Part model, mm, in its own coordinate system. Round coordinates to 2 decimals unless told otherwise and drop trailing zeros. Write each loop counter-clockwise with the first axis right and the second up, starting at its lowest first coordinate (ties: lowest second). Pieces come first, ordered by that corner, then holes. Notation, with made-up numbers: (-19.75, -31) -> (28.25, -31) arc R15 ccw to (28.25, -16) -> close; hole circle Ø10 at (82.5, -6.75). An arc over 180 degrees is marked (long way). Use CSV: the item, a comma, the result in double quotes. Start each with the question number.
(1) Probe line 1 (Z direction, x = 17.5, y = 41); line 2 (Y direction, x = 14.5, z = 15); line 3 (Y direction, x = 12.25, z = 35). List the from-to ranges inside material, lowest first. Write a range as [from, to].
(2) Saw through at D-D (y = 30.5). Give the cut face in (x, z).
(3) Saw through at C-C (y = 42.5). Count the separate pieces of the cut face and the enclosed holes in it, plus the area to 3 significant figures.
(4) Two-plate mould, pull along Z, no slides. Class faces 1 (the flat face through (10, 65, 25)), 2 (the flat face through (12, 33, 0)), 3 (the cylindrical face through (9.63, 44.47, 15.52)): released by +Z, released by -Z, zero draft, split by the parting line, or undercut.
(5) Saw through at B-B (z = 41.5). Give the cut face in (x, y), plus the area to 3 significant figures.
(6) Saw through at A-A (z = 15). Give the cut face in (x, y).
(7) Drop flat-ended pins along their axis: pin 1 (4 mm diameter, centred on y = 57, z = 27.5, fed in from -X); pin 2 (1 mm diameter, centred on y = 29, z = 18, fed in from -X). Give the stop position or say it passes through.
```python
from build123d import *

# Parameters (mm, degrees)
BOSS_EXTRUDE1_DEPTH = 50
SKETCH2_R           = 4
CUT_EXTRUDE1_DEPTH  = 20
CHAMFER1_SIZE       = 1


with BuildPart() as part:
    # Sketch1 → Boss-Extrude1 (new body)
    with BuildSketch(Plane.XY):
        with BuildLine():
            Line((0, 0), (20, 0))
            Line((20, 0), (20, 65))
            Line((20, 65), (0, 65))
            Line((0, 65), (0, 61.14955156))
            ThreePointArc((0, 61.14955156), (6.5, 53.716517187), (0, 46.283482813))
            Line((0, 46.283482813), (0, 33.716517187))
            ThreePointArc((0, 33.716517187), (14, 18.74988764), (0, 3.783258093))
            Line((0, 3.783258093), (0, 0))
        make_face()
    extrude(amount=BOSS_EXTRUDE1_DEPTH)

    # Sketch2 → Cut-Extrude1 (cut)
    with BuildSketch(Plane(origin=(20, 0, 0), x_dir=(0, 0, -1), z_dir=(1, 0, 0))):
        with Locations((-35, 40.505102572)):
            Circle(SKETCH2_R)
        with Locations((-15, 40.505102572)):
            Circle(SKETCH2_R)
    extrude(amount=-CUT_EXTRUDE1_DEPTH, mode=Mode.SUBTRACT)

    # Chamfer1
    chamfer1_edges = [part.edges().sort_by_distance(p)[0] for p in [
        (20, 40.505102572, 39),
        (20, 40.505102572, 19),
    ]]
    chamfer(chamfer1_edges, length=CHAMFER1_SIZE)


solid = part.part
```
Answers:
1,line 1,"z = [0, 11.03], [18.97, 31.03], [38.97, 50]"
1,line 2,"y = [0, 36.51], [44.51, 65]"
1,line 3,"y = [0, 11.72], [25.78, 36.51], [44.51, 65]"
2,outline,"(8.32, 0) -> (20, 0) -> (20, 50) -> (8.32, 50) -> close"
3,separate pieces,"3"
3,enclosed holes,"0"
3,area,"720 mm²"
4,face 1,"zero draft"
4,face 2,"released by -Z"
4,face 3,"undercut"
5,outline,"(0, 0) -> (20, 0) -> (20, 65) -> (0, 65) -> (0, 61.15) arc R7.5 cw to (0, 46.28) -> (0, 33.72) arc R15 cw to (0, 3.78) -> close"
5,area,"903 mm²"
6,outline,"(0, 0) -> (20, 0) -> (20, 35.51) -> (19, 36.51) -> (0, 36.51) -> (0, 33.72) arc R15 cw to (0, 3.78) -> close; (0, 44.51) -> (19, 44.51) -> (20, 45.51) -> (20, 65) -> (0, 65) -> (0, 61.15) arc R7.5 cw to (0, 46.28) -> close"
7,pin 1,"stops at x = 4.32"
7,pin 2,"stops at x = 9.46"
